Geometry: final body of the model. Coordinates: model frame, mm. Face numbers are marked on the shaded views. Round coordinates to 2 decimals unless told otherwise and drop trailing zeros. Loops run counter-clockwise (first coordinate to the right, second up) from the corner with the lowest first, then second, coordinate; pieces in that order, holes last. Notation, with made-up numbers: (42, -15) - (83, -15) arc R25 ccw to (83, 2) - close; hole circle Ø11 at (23, 0). An arc over 180 degrees is marked (long way). Use CSV: the item, a comma, the result in double quotes.
from build123d import *

# Parameters (mm, degrees)
SKETCH1_W           = 110
SKETCH1_H           = 110
BOSS_EXTRUDE1_DEPTH = 6
FILLET1_R           = 10
SKETCH12_R          = 5
BOSS_EXTRUDE5_DEPTH = 12
SKETCH13_R          = 5
BOSS_EXTRUDE6_DEPTH = 12
SKETCH14_R          = 5
BOSS_EXTRUDE7_DEPTH = 12
SKETCH15_R          = 5
BOSS_EXTRUDE8_DEPTH = 12


with BuildPart() as part:
    # Sketch1 → Boss-Extrude1 (new body)
    with BuildSketch(Plane(origin=(0, 0, 0), x_dir=(1, 0, 0), z_dir=(0, 1, 0))):
        with Locations((55, 55)):
            Rectangle(SKETCH1_W, SKETCH1_H)
    extrude(amount=BOSS_EXTRUDE1_DEPTH)

    # Fillet1
    fillet1_edges = [part.edges().sort_by_distance(p)[0] for p in [
        (0, 3, -110),
        (110, 3, -110),
        (110, 3, 0),
        (0, 3, 0),
    ]]
    fillet(fillet1_edges, radius=FILLET1_R)

    # Sketch12 → Boss-Extrude5 (add)
    with BuildSketch(Plane(origin=(0, 6, 0), x_dir=(1, 0, 0), z_dir=(0, 1, 0))):
        with Locations(Location((39, 16, 0), (0, 0, 90))):
            Circle(SKETCH12_R)
    extrude(amount=BOSS_EXTRUDE5_DEPTH)

    # Sketch13 → Boss-Extrude6 (add)
    with BuildSketch(Plane(origin=(0, 6, 0), x_dir=(1, 0, 0), z_dir=(0, 1, 0))):
        with Locations(Location((71, 16, 0), (0, 0, 90))):
            Circle(SKETCH13_R)
    extrude(amount=BOSS_EXTRUDE6_DEPTH)

    # Sketch14 → Boss-Extrude7 (add)
    with BuildSketch(Plane(origin=(0, 6, 0), x_dir=(1, 0, 0), z_dir=(0, 1, 0))):
        with Locations(Location((10, 10, 0), (0, 0, 90))):
            Circle(SKETCH14_R)
    extrude(amount=BOSS_EXTRUDE7_DEPTH)

    # Sketch15 → Boss-Extrude8 (add)
    with BuildSketch(Plane(origin=(0, 6, 0), x_dir=(1, 0, 0), z_dir=(0, 1, 0))):
        with Locations(Location((100, 10, 0), (0, 0, 90))):
            Circle(SKETCH15_R)
    extrude(amount=BOSS_EXTRUDE8_DEPTH)


solid = part.part
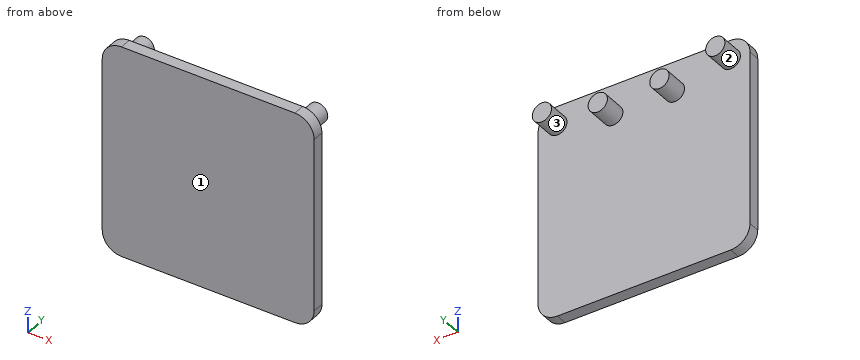
Item 1: Material intervals for line 1 (Y direction, x = 13, z = -59); line 2 (Z direction, x = 99.5, y = 16.75); line 3 (X direction, y = 16.75, z = -18.5), sorted ascending.
Final values:
line 1,"y = 0 to 6"
line 2,"z = -14.97 to -5.03"
line 3,"x = 34.67 to 43.33, 66.67 to 75.33"
Item 2: Mould query, pull axis X, two halves, no side actions, for the marked faces 1, 2 and 3. Classes: released by +X, released by -X, zero draft, split by the parting line, or undercut.
Final values:
face 1,"zero draft"
face 2,"undercut"
face 3,"undercut"
Item 3: Section A-A on x = 39. Return the cut outline in (y, z), plus the area to 3 significant figures.
Final values:
outline,"(0, -110) - (6, -110) - (6, -21) - (18, -21) - (18, -11) - (6, -11) - (6, 0) - (0, 0) - close"
area,"780 mm²"
Item 4: Section C-C on y = 11.75. Return the cut outline in (x, z), plus the area to 3 significant figures.
Final values:
outline,"circle Ø10 at (10, -10); circle Ø10 at (39, -16); circle Ø10 at (71, -16); circle Ø10 at (100, -10)"
area,"314 mm²"
Item 5: Section D-D on z = -41. Return the cut outline in (x, y), plus the area to 3 significant figures.
Final values:
outline,"(0, 0) - (110, 0) - (110, 6) - (0, 6) - close"
area,"660 mm²"
Item 6: Section B-B on z = -13. Return the cut outline in (x, y), plus the area to 3 significant figures.
Final values:
outline,"(0, 0) - (110, 0) - (110, 6) - (104, 6) - (104, 18) - (96, 18) - (96, 6) - (75, 6) - (75, 18) - (67, 18) - (67, 6) - (43, 6) - (43, 18) - (35, 18) - (35, 6) - (14, 6) - (14, 18) - (6, 18) - (6, 6) - (0, 6) - close"
area,"1,040 mm²"
